For this review, take the finished solid that the model builds, in its own axes (mm). A direction names the side the tool comes from. Round coordinates to 2 decimals unless told otherwise and drop trailing zeros. Order: outer loops, then holes, each group sorted by start corner. A loop starts at its lowest first (then second) coordinate and runs counter-clockwise, first axis right, second up. Notation, with made-up numbers: M -29.75,43 L -6.75,43 A13 ccw -6.75,53 Z; hole C 42,-0.5 d10. An arc over 180 degrees is marked long. Answer in a Markdown table with one row per item. Add a question column.
```python
from build123d import *

# Parameters (mm, degrees)
SKETCH1_W           = 54
SKETCH1_H           = 20
SKETCH1_W_2         = 2.54
SKETCH1_H_2         = 3
BOSS_EXTRUDE1_DEPTH = 5


with BuildPart() as part:
    # Sketch1 → Boss-Extrude1 (new body)
    with BuildSketch(Plane(origin=(0, 0, 0), x_dir=(1, 0, 0), z_dir=(0, 1, 0))):
        Rectangle(SKETCH1_W, SKETCH1_H)
        with Locations((-16.962, -11.5)):
            Rectangle(SKETCH1_W_2, SKETCH1_H_2)
        with Locations((-5.654, -11.5)):
            Rectangle(SKETCH1_W_2, SKETCH1_H_2)
        with Locations((5.654, -11.5)):
            Rectangle(SKETCH1_W_2, SKETCH1_H_2)
        with Locations((16.962, -11.5)):
            Rectangle(SKETCH1_W_2, SKETCH1_H_2)
        with Locations((16.962, 11.5)):
            Rectangle(SKETCH1_W_2, SKETCH1_H_2)
        with Locations((5.654, 11.5)):
            Rectangle(SKETCH1_W_2, SKETCH1_H_2)
        with Locations((-5.654, 11.5)):
            Rectangle(SKETCH1_W_2, SKETCH1_H_2)
        with Locations((-16.962, 11.5)):
            Rectangle(SKETCH1_W_2, SKETCH1_H_2)
    extrude(amount=BOSS_EXTRUDE1_DEPTH)


solid = part.part
```
1. For faces 4 (the flat face through (18.232, 2, -11)), 5 (the flat face through (6.924, 2, 12)), 6 (the flat face through (-18.232, 2, 12)), 7 (the flat face through (-15.692, 2, -11)), list the 3-axis set-ups (+Z, -Z, +X, -X, +Y, -Y) from which the entire face can be reached by the end or side of a thin tool; tool diameter is ignored.
2. Consider section A-A on z = 10.5. Write out the cut boundary in (x, y), plus the area to 3 significant figures.
3. The part is to be moulded in two halves that separate along X. For faces 1 (the flat face through (4.384, 2, -11)), 2 (the flat face through (18.232, 2, 12)), 3 (the flat face through (-6, 2, 13)), say which applies: pulls with the +X half, pulls with the -X half, needs draft (parallel to the pull), parting line crosses it, or undercut.
4. Clearance check with flat-ended pins moving along their axes: pin 1 Ø1.5 at (y, z) = (3, 11) entering from +X; pin 2 Ø1.5 at (y, z) = (3, 11.5) entering from -X; pin 3 Ø1.5 at (x, y) = (9.5, 2.5) entering from -Z. State where each tip first meets the part, or that it passes through.
5. Consider section B-B on x = 9.5. Write out the cut boundary in (y, z), plus the area to 3 significant figures.
6. To check wall thickness, follow probe 1 along Z at (x, y) = (-2, 2.9). State the ranges of the line that lie inside material, in increasing order. Write a range as [from, to].
Solved:
| question | item | result |
|---|---|---|
| 1 | face 4 | -Z, +X, +Y, -Y |
| 1 | face 5 | +Z, +Y, -Y |
| 1 | face 6 | +Z, -X, +Y, -Y |
| 1 | face 7 | -Z, +Y, -Y |
| 2 | outline | M -18.23,0 L -15.69,0 L -15.69,5 L -18.23,5 Z; M -6.92,0 L -4.38,0 L -4.38,5 L -6.92,5 Z; M 4.38,0 L 6.92,0 L 6.92,5 L 4.38,5 Z; M 15.69,0 L 18.23,0 L 18.23,5 L 15.69,5 Z |
| 2 | area | 50.8 mm^2 |
| 3 | face 1 | undercut |
| 3 | face 2 | pulls with the +X half |
| 3 | face 3 | needs draft |
| 4 | pin 1 | stops at x = 18.23 |
| 4 | pin 2 | stops at x = -18.23 |
| 4 | pin 3 | stops at z = -10 |
| 5 | outline | M 0,-10 L 5,-10 L 5,10 L 0,10 Z |
| 5 | area | 100 mm^2 |
| 6 | probe 1 | z = [-10, 10] |
